Can you work these out from the model? Positions are in its coordinate system, mm. A direction names the side the tool comes from. Give positions to 0.01 mm unless a question says otherwise; leave off trailing zeros. Order: outer loops, then holes, each group sorted by start corner. A loop starts at its lowest first (then second) coordinate and runs counter-clockwise, first axis right, second up. Notation, with made-up numbers: M 57,-30.5 L 64,-30.5 A23 cw 64,-1.5 Z; hole C -30.75,29 d5. An arc over 180 degrees is marked long. Use one line per item in the form item = value. Start each with the question number.
1. I need wall thicknesses on L1, parallel to Y at x = 0, z = 73; L2, parallel to X at y = 18.5, z = 49; L3, parallel to X at y = -12.5, z = 11. Which ranges of each line are inside material? Lowest first, please.
2. Will these pins go through, and if not, where does the flat tip stop? P1, Ø2, axis at y = -37.5, z = 45, coming from the +X side; P2, Ø2, axis at y = -43, z = 25.5, coming from the -X side; P3, Ø22, axis at x = 208, z = 33.5, coming from the +Y side.
3. I want a section at B-B, the plane x = 0. List the corners of the cut face in (y, z) for me, and give its area (3 significant figures).
4. For faces 3 (the face through (95.88, 47.26, 46.49)), 4 (the face through (-3.31, 25.23, 45.21)), 5 (the face through (219.07, -44.93, 46.49)), which set-ups out of +Z, -Z, +X, -X, +Y, -Y let a thin tool reach every point of the face, with its end or its side?
5. I want a section at C-C, the plane y = -9.5. List the corners of the cut face in (x, z) for me.
6. I want a section at D-D, the plane x = 261.5. List the corners of the cut face in (y, z) for me, and give its area (3 significant figures).
7. I want a section at A-A, the plane z = 7.5. List the corners of the cut face in (x, y) for me (3 decimals).
8. We'd pull the mould along X, two halves only. Please class faces 1 (the face through (221, 43.201, 45)), 2 (the face through (135, 1, 91.702)): +X half, -X half, draft (parallel to the pull), parting line (faces both ways), or undercut.
```python
from build123d import *

# Parameters (mm, degrees)
F0_R     = 25.444736
F1_DEPTH = 91.702167
F2_R     = 959.987855


with BuildPart() as f1:
    # F0 (on Top) → F1 (new body)
    with BuildSketch(Plane.XY):
        with BuildLine():
            ThreePointArc((41.567442, 43.200706), (55.16418, 23.474804), (59.951257, 0))
            Line((59.951257, 0), (233.576013, 0))
            ThreePointArc((233.576013, 0), (240.029875, 24.751712), (257.748065, 43.200706))
            Line((257.748065, 43.200706), (41.567442, 43.200706))
        make_face()
        with BuildLine():
            ThreePointArc((257.748065, 43.200706), (240.029875, 24.751712), (233.576013, 0))
            ThreePointArc((233.576013, 0), (240.029875, -24.751712), (257.748065, -43.200706))
            ThreePointArc((257.748065, -43.200706), (309.018274, -44.236686), (334.957109, 0))
            ThreePointArc((334.957109, 0), (309.018274, 44.236686), (257.748065, 43.200706))
        make_face()
        with BuildLine():
            ThreePointArc((314.711569, 0), (284.266561, -30.445007), (253.821554, 0))
            ThreePointArc((253.821554, 0), (284.266561, 30.445007), (314.711569, 0))
        make_face(mode=Mode.SUBTRACT)
        with BuildLine():
            Line((233.576013, 0), (59.951257, 0))
            ThreePointArc((59.951257, 0), (55.16418, -23.474804), (41.567442, -43.200706))
            Line((41.567442, -43.200706), (257.748065, -43.200706))
            ThreePointArc((257.748065, -43.200706), (240.029875, -24.751712), (233.576013, 0))
        make_face()
        with BuildLine():
            ThreePointArc((41.567442, -43.200706), (55.16418, -23.474804), (59.951257, 0))
            ThreePointArc((59.951257, 0), (55.16418, 23.474804), (41.567442, 43.200706))
            ThreePointArc((41.567442, 43.200706), (-59.951257, 0), (41.567442, -43.200706))
        make_face()
        Circle(F0_R, mode=Mode.SUBTRACT)
    extrude(amount=F1_DEPTH)

    # F2
    f2_edges = [f1.edges().sort_by_distance(p)[0] for p in [
        (257.748065, -43.200706, 45.851083),
        (41.567442, 43.200706, 45.851083),
    ]]
    fillet(f2_edges, radius=F2_R)


solid = f1.part
```
Check result:
q1.L1 = -59.95 to -25.44, 25.44 to 59.95
q1.L2 = -57.03 to -17.47, 17.47 to 260.09, 308.45 to 331.46
q1.L3 = -58.63 to -22.16, 22.16 to 256.51, 312.03 to 333.39
q2.P1 = 319.44
q2.P2 = -42.78
q2.P3 = 43.2
q3.outline = M -59.95,0 L -25.44,0 L -25.44,91.7 L -59.95,91.7 Z; M 25.44,0 L 59.95,0 L 59.95,91.7 L 25.44,91.7 Z
q3.area = 6,330 mm2
q4.face_3 = +Z, -Z, +Y
q4.face_4 = +Z, -Z
q4.face_5 = +Z, -Z, -Y
q5.outline = M -59.19,0 L -23.6,0 L -23.6,91.7 L -59.19,91.7 Z; M 23.6,0 L 255.34,0 L 255.34,91.7 L 23.6,91.7 Z; M 313.19,0 L 334.06,0 L 334.06,91.7 L 313.19,91.7 Z
q6.outline = M -48.43,0 L -20.21,0 L -20.21,91.7 L -48.43,91.7 Z; M 20.21,0 L 45.29,0 L 45.29,91.7 L 20.21,91.7 Z
q6.area = 4,890 mm2
q7.outline = M 10.821,58.967 A59.951 ccw long 41.567,-43.201 L 161.451,-43.201 A959.988 cw 278.107,-50.315 A50.691 ccw 334.957,0 A50.691 ccw 257.748,43.201 L 184.088,43.201 A959.988 cw Z; hole C 0,0 d50.889; hole C 284.267,0 d60.89
q8.face_1 = undercut
q8.face_2 = draft
